Build history of the part. All positions in model axes, mm. Round coordinates to 2 decimals unless told otherwise and drop trailing zeros. Loops run counter-clockwise (first coordinate to the right, second up) from the corner with the lowest first, then second, coordinate; pieces in that order, holes last. Notation, with made-up numbers: (61, -39) - (96, -39) arc R19 ccw to (96, -8) - close; hole circle Ø6 at (7.5, 13.5). An arc over 180 degrees is marked (long way). Put each result on its own line as item: value. Start each with the question number.
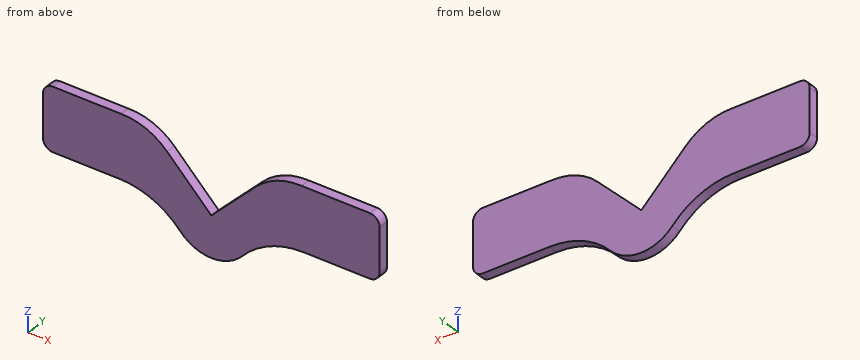
from build123d import *

# Parameters (mm, degrees)
F1_DEPTH = 3


with BuildPart() as f1:
    # F0 (on Front) → F1 (new body)
    with BuildSketch(Plane.XZ):
        with BuildLine():
            ThreePointArc((-48, -22.5), (-50.12132, -23.37868), (-51, -25.5))
            Line((-51, -25.5), (-51, -38.5))
            ThreePointArc((-51, -38.5), (-50.12132, -40.62132), (-48, -41.5))
            Line((-48, -41.5), (-27.869387, -41.5))
            ThreePointArc((-27.869387, -41.5), (-17.767422, -43.631894), (-9.388361, -49.663977))
            ThreePointArc((-9.388361, -49.663977), (0, -53.811277), (9.388361, -49.663977))
            ThreePointArc((9.388361, -49.663977), (17.767422, -43.631894), (27.869387, -41.5))
            Line((27.869387, -41.5), (0, -41.5))
            Line((0, -41.5), (-13.44061, -28.05939))
            ThreePointArc((-13.44061, -28.05939), (-19.817915, -23.853882), (-27.336115, -22.5))
            Line((-27.336115, -22.5), (-48, -22.5))
        make_face()
        with BuildLine():
            Line((13.44061, -28.05939), (0, -41.5))
            Line((0, -41.5), (27.869387, -41.5))
            Line((27.869387, -41.5), (48, -41.5))
            ThreePointArc((48, -41.5), (50.12132, -40.62132), (51, -38.5))
            Line((51, -38.5), (51, -25.5))
            ThreePointArc((51, -25.5), (50.12132, -23.37868), (48, -22.5))
            Line((48, -22.5), (27.336115, -22.5))
            ThreePointArc((27.336115, -22.5), (19.817915, -23.853882), (13.44061, -28.05939))
        make_face()
    extrude(amount=F1_DEPTH)


solid = f1.part
Item 1: Slice it at D-D (x = -41). Give the cut face in (y, z), plus the area to 3 significant figures.
Item 2: Drill centre lines: probe 1 along Z at (x, y) = (37, -1.95); probe 2 along X at (y, z) = (-1.4, -31); probe 3 along X at (y, z) = (-2.4, -26). Where is each one in solid material? Low to high. Write a range as [from, to].
Item 3: Slice it at A-A (z = -37.5). Give the cut face in (x, y).
Item 4: Slice it at C-C (y = -0.85). Give the cut face in (x, z).
Item 5: Slice it at B-B (z = -30). Give the cut face in (x, y).
Item 6: Drop flat-ended pins along their axis: pin 1 Ø1.5 at (x, y) = (35, -1.5) entering from -Z; pin 2 Ø1.5 at (x, y) = (35, -1) entering from +Z; pin 3 Ø1.5 at (y, z) = (-1, -50.5) entering from +X. Give the stop position or say it passes through.
Computed values:
1. outline: (-3, -41.5) - (0, -41.5) - (0, -22.5) - (-3, -22.5) - close
1. area: 57.0 mm^2
2. probe 1: z = [-41.5, -22.5]
2. probe 2: x = [-51, -10.5], [10.5, 51]
2. probe 3: x = [-51, -15.88], [15.88, 51]
3. outline: (-51, -3) - (-4, -3) - (-4, 0) - (-51, 0) - close; (4, -3) - (51, -3) - (51, 0) - (4, 0) - close
4. outline: (-51, -38.5) arc R3 ccw to (-48, -41.5) - (-27.87, -41.5) arc R25 cw to (-9.39, -49.66) arc R12.7 ccw to (9.39, -49.66) arc R25 cw to (27.87, -41.5) - (48, -41.5) arc R3 ccw to (51, -38.5) - (51, -25.5) arc R3 ccw to (48, -22.5) - (27.34, -22.5) arc R19 ccw to (13.44, -28.06) - (0, -41.5) - (-13.44, -28.06) arc R19 ccw to (-27.34, -22.5) - (-48, -22.5) arc R3 ccw to (-51, -25.5) - close
5. outline: (-51, -3) - (-11.5, -3) - (-11.5, 0) - (-51, 0) - close; (11.5, -3) - (51, -3) - (51, 0) - (11.5, 0) - close
6. pin 1: stops at z = -41.5
6. pin 2: stops at z = -22.5
6. pin 3: stops at x = 9.31
